Autodesk Inventor part; units mm, degrees
ref_plane "YZ Plane" through (0, 0, 0) normal (1, 0, 0) x (0, 1, 0)
ref_plane "XZ Plane" through (0, 0, 0) normal (0, 1, 0) x (-1, 0, 0)
ref_plane "XY Plane" through (0, 0, 0) normal (0, 0, 1) x (1, 0, 0)
sketch "Sketch1" plane through (0, 0, 0) normal (0, 0, 1) x (1, 0, 0)
  circle A0 centre (0, 0) radius 30
  line L0 (50, -50) -> (-50, -50)
  line L1 (-50, -50) -> (-50, 50)
  line L2 (-50, 50) -> (50, 50)
  line L3 (50, 50) -> (50, -50)
  line L4 (50, -50) -> (-50, 50) construction
  line L5 (-50, -50) -> (50, 50) construction
  dimension "d2" = 60
  dimension "d30" = 100
  dimension "d31" = 100
extrude "Extrusion1" add sketch "Sketch1" along normal blind 10 contours A0 | L0 L1 L2 L3
sketch "Sketch2" plane through (0, 0, 0) normal (0, 0, -1) x (-1, 0, 0)
  circle A0 centre (0, 0) radius 25 construction
  line L0 (0, 0) -> (-12.5, 21.6506) construction
  line L1 (0, 0) -> (25, 0) construction
  line L2 (0, 0) -> (-25, 0) construction
  line L3 (0, 0) -> (12.5, -21.6506) construction
  line L4 (0, 0) -> (12.5, 21.6506) construction
  line L5 (0, 0) -> (-12.5, -21.6506) construction
  circle A1 centre (12.5, 21.6506) radius 2.5
  circle A2 centre (-12.5, 21.6506) radius 2.5
  circle A3 centre (-25, 0) radius 2.5
  circle A4 centre (-12.5, -21.6506) radius 2.5
  circle A5 centre (12.5, -21.6506) radius 2.5
  circle A6 centre (25, 0) radius 2.5
  dimension "d3" = 50
  dimension "d4" = 60
  dimension "d5" = 60
  dimension "d6" = 60
  dimension "d7" = 60
  dimension "d8" = 60
  dimension "d9" = 5
  dimension "d10" = 5
  dimension "d11" = 5
  dimension "d12" = 5
  dimension "d13" = 5
  dimension "d14" = 5
extrude "Extrusion2" cut sketch "Sketch2" against normal through all
sketch "Sketch8" plane through (0, 0, 0) normal (0, 0, -1) x (-1, 0, 0)
  circle A0 centre (0, 0) radius 30
  circle A1 centre (-12.5, 21.6506) radius 2.5
  circle A2 centre (-25, 0) radius 2.5
  circle A3 centre (-12.5, -21.6506) radius 2.5
  circle A4 centre (12.5, -21.6506) radius 2.5
  circle A5 centre (25, 0) radius 2.5
  circle A6 centre (12.5, 21.6506) radius 2.5
  dimension "d34" = 60
extrude "Extrusion5" add sketch "Sketch8" against normal blind 11
sketch "Sketch9" plane through (0, 0, 10) normal (0, 0, 1) x (1, 0, 0)
  circle A0 centre (0, 0) radius 30
  line L0 (50, 50) -> (-50, 50)
  line L1 (-50, 50) -> (-50, -50)
  line L2 (-50, -50) -> (50, -50)
  line L3 (50, -50) -> (50, 50)
  line L4 (-45, -45) -> (-45, 45)
  line L5 (-45, 45) -> (45, 45)
  line L6 (45, 45) -> (45, -45)
  line L7 (45, -45) -> (-45, -45)
  dimension "d37" = 5
extrude "Extrusion6" add sketch "Sketch9" along normal blind 40 contours L3 L2 L1 L0
sketch "Sketch10" plane through (0, 0, 50) normal (0, 0, 1) x (1, 0, 0)
  circle A0 centre (0, 0) radius 20.5
  dimension "d40" = 41
sketch "Sketch11" plane through (0, 0, 0) normal (0, 1, 0) x (-1, 0, 0)
  line L0 (45, 50) -> (-45, 50)
  line L1 (0, 50) -> (0, 55)
  line L2 (-50, 50) -> (50, 50)
  line L3 (-20.5, 55) -> (20.5, 55)
  arc A0 (20.5, 55) -> (50, 50) centre (50, 139.525) ccw
  arc A1 (-50, 50) -> (-20.5, 55) centre (-50, 139.525) ccw
  line L4 (20.5, 55) -> (20.5, 50)
  line L5 (20.5, 50) -> (20.5, 45)
  line L6 (20.5, 45) -> (50, 45)
  line L7 (50, 45) -> (50, 50)
  point P0 (0, 0)
  dimension "d41" = 5
  dimension "d42" = 41
  dimension "d43" = 5
revolve "Revolution2" add sketch "Sketch11" angle 360 about axis through (0, 0, 50) along (0, 0, 1) contours L2 L7 L6 L5 L0 | L0 L4 A0 L2
sketch "Sketch12" plane through (0, 0, 50) normal (0, 0, 1) x (1, 0, 0)
  arc A0 (-21.7945, 45) -> (-45, 21.7945) centre (0, 0) ccw
  line L0 (-45, -45) -> (45, -45)
  line L1 (45, -45) -> (45, 45)
  line L2 (45, 45) -> (-45, 45)
  line L3 (-45, 45) -> (-45, -45)
  circle A1 centre (0, 0) radius 30
  arc A2 (45, 21.7945) -> (21.7945, 45) centre (0, 0) ccw
  arc A3 (21.7945, -45) -> (45, -21.7945) centre (0, 0) ccw
  arc A4 (-45, -21.7945) -> (-21.7945, -45) centre (0, 0) ccw
  point P0 (-45, 21.7945)
  point P1 (-21.7945, 45)
extrude "Extrusion7" add sketch "Sketch12" against normal blind 5 contours A0 L3 L2 | L2 L1 A2 | A4 L0 L3 | L1 L0 A3
sketch "Sketch13" plane through (0, 0, 0) normal (0, 1, 0) x (-1, 0, 0)
  line L0 (45, 10) -> (45, 45)
  line L1 (45, 10) -> (50, 10)
  line L2 (50, 0) -> (50, 50)
  line L3 (50, 10) -> (50, 79.5964)
  line L4 (50, 79.5964) -> (-50, 79.5964)
  line L5 (-45, 10) -> (-45, 45)
  line L6 (-45, 10) -> (-50, 10)
  line L7 (-50, 0) -> (-50, 50)
  line L8 (-50, 10) -> (-50, 79.5964)
  line L9 (-45, 10) -> (45, 10)
  line L10 (30, 11) -> (-30, 11)
  line L11 (30, 10) -> (30, 11)
  line L12 (-30, 10) -> (-30, 11)
  point P0 (0, 0)
  dimension "d47" = 100
extrude "Extrusion8" cut sketch "Sketch13" against normal through all contours L9 L11 L10 L12 L6 L7 L8 L4 L3 L2 L1
sketch "Sketch14" plane through (-50, -50, 0) normal (0, -1, 0) x (1, 0, 0)
  line L0 (80, 11) -> (20, 11)
  line L1 (100, 10) -> (80, 10)
  line L2 (20, 11) -> (80, 11)
  line L3 (80, 11) -> (80, 10)
  line L4 (80, 10) -> (20, 10)
  line L5 (20, 10) -> (20, 11)
  point P0 (50, 0)
extrude "Extrusion9" cut sketch "Sketch14" against normal blind 10
properties part number "soporte"
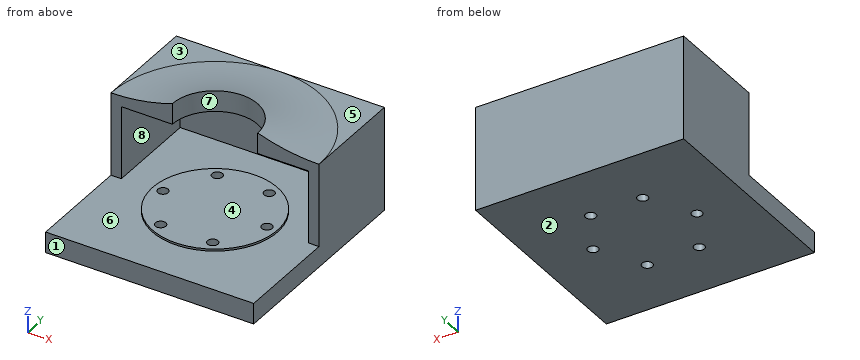
The listing builds one solid part. Answer for the finished solid, in the listing's coordinates (mm). Face numbers are marked on the shaded views. A direction names the side the tool comes from. Round coordinates to 2 decimals unless told otherwise and drop trailing zeros. Loops run counter-clockwise (first coordinate to the right, second up) from the corner with the lowest first, then second, coordinate; pieces in that order, holes last. Notation, with made-up numbers: (62, 81) -> (86, 81) arc R27 cw to (86, 105) -> close; hole circle Ø2 at (30.25, -38.75). An arc over 180 degrees is marked (long way). Use one line per item in the form item = value.
1. The part is cut by section B-B on x = -12.5. Give the number of separate pieces and of enclosed holes in the cut face, and give its area (3 significant figures).
Answer key:
separate_pieces = 3
enclosed_holes = 0
area = 1,340 mm²
2. The part is cut by section A-A on z = 24. Determine the outline of the cut face in (x, y).
Answer key:
outline = (-50, 0) -> (-45, 0) -> (-45, 45) -> (45, 45) -> (45, 0) -> (50, 0) -> (50, 50) -> (-50, 50) -> close
3. Flat-ended cylindrical pins translate along their axes: pin 1 Ø15 at (x, y) = (17.5, 24.5) entering from +Z; pin 2 Ø3 at (x, z) = (6, 46.5) entering from -Y; pin 3 Ø6 at (x, y) = (12.5, -21.65) entering from -Z; pin 4 Ø4 at (x, z) = (8, 26.5) entering from -Y. Find the tip coordinate at first contact, or state that the pin passes through.
Answer key:
pin_1 = 54.29
pin_2 = 19.08
pin_3 = 0
pin_4 = 45
4. Find the intervals of material crossed by probe 1 along Y at (x, z) = (-12.5, 6.5); probe 2 along Y at (x, z) = (25, 8); probe 3 along X at (y, z) = (44, 24), in increasing order. Write a range as [from, to].
Answer key:
probe_1 = [-50, -24.15], [-19.15, 19.15], [24.15, 50]
probe_2 = [-50, -2.5], [2.5, 50]
probe_3 = [-50, -45], [45, 50]
5. A tool of negligible diameter and unlimited length cuts with its end or side. For the marked faces 5, 6, 7 and 8, from which of +Z, -Z, +X, -X, +Y, -Y can it reach the whole face along a straight path? Write none if from no direction.
Answer key:
face_5 = +Z, +X, +Y
face_6 = none
face_7 = +Z, -Y
face_8 = -Y
6. For a pull along Z with two mould halves and no side action, classify the marked faces 1, 2, 3 and 4 as released by +Z, released by -Z, zero draft, split by the parting line, or undercut.
Answer key:
face_1 = zero draft
face_2 = released by -Z
face_3 = released by +Z
face_4 = undercut
